Check sheet for the modelled part. Datum: model origin and axes. Units: mm. A direction names the side the tool comes from. Give positions to 0.01 mm unless a question says otherwise; leave off trailing zeros. Order: outer loops, then holes, each group sorted by start corner. A loop starts at its lowest first (then second) coordinate and runs counter-clockwise, first axis right, second up.
```python
from build123d import *

# Parameters (mm, degrees)
SKETCH_R      = 19
SKETCH_R_2    = 4
PAD_DEPTH     = 2
SKETCH001_R   = 15
SKETCH001_R_2 = 4
PAD001_DEPTH  = 1.4
SKETCH002_W   = 8.5
SKETCH002_H   = 8.5
POCKET_DEPTH  = 6


with BuildPart() as part:
    # Sketch → Pad (new body)
    with BuildSketch(Plane.XY):
        Circle(SKETCH_R)
        Circle(SKETCH_R_2, mode=Mode.SUBTRACT)
    extrude(amount=PAD_DEPTH)

    # Sketch001 (on Face4 of Pad) → Pad001 (join)
    with BuildSketch(Plane.XY.offset(2)):
        Circle(SKETCH001_R)
        Circle(SKETCH001_R_2, mode=Mode.SUBTRACT)
    extrude(amount=PAD001_DEPTH)

    # Sketch002 (on Face7 of Pad001) → Pocket (cut)
    with BuildSketch(Plane.XY.offset(3.4)):
        Rectangle(SKETCH002_W, SKETCH002_H)
    extrude(amount=-POCKET_DEPTH, mode=Mode.SUBTRACT)


solid = part.part
```
(1) Cross-section at D-D on x = 7.5. Enter the section's corners in (y, z), then the cut area to 3 significant figures.
Response values:
outline: (-17.46, 0) - (17.46, 0) - (17.46, 2) - (12.99, 2) - (12.99, 3.4) - (-12.99, 3.4) - (-12.99, 2) - (-17.46, 2) - close
area: 106 mm2
(2) Set-up check for faces 1 (the face through (-14.985, 0.66, 2.69)), 2 (the face through (-0.3, 4.5, 0)), 3 (the face through (4.25, 0, 2)): record each of +Z, -Z, +X, -X, +Y, -Y from which the full face is reachable in a straight line by a thin tool's end or side.
Response values:
face 1: +Z
face 2: -Z, +X, -X, +Y, -Y
face 3: +Z, -Z
(3) Cross-section at A-A on y = 0. Enter the section's corners in (x, z), then the cut area to 3 significant figures.
Response values:
outline: (-19, 0) - (-4.25, 0) - (-4.25, 3.4) - (-15, 3.4) - (-15, 2) - (-19, 2) - close; (4.25, 0) - (19, 0) - (19, 2) - (15, 2) - (15, 3.4) - (4.25, 3.4) - close
area: 89.1 mm2
(4) Material ranges on L1, parallel to X at y = 0.5, z = 0.7; L2, parallel to X at y = 3, z = 1; L3, parallel to Z at x = -17, y = 6, recorded low to high.
Response values:
L1: x = -18.99 to -4.25, 4.25 to 18.99
L2: x = -18.76 to -4.25, 4.25 to 18.76
L3: z = 0 to 2
(5) Cross-section at C-C on z = 0.7. Enter the section's corners in (x, y), then the cut area to 3 significant figures.
Response values:
outline: circle Ø38 at (0, 0); hole (-4.25, -4.25) - (4.25, -4.25) - (4.25, 4.25) - (-4.25, 4.25) - close
area: 1,060 mm2
(6) Release check for a two-part mould opening along X. For faces 4 (the face through (8.767, -16.856, 0.986)), 5 (the face through (-4.25, 0, 2)), 6 (the face through (14, 6, 2)), 7 (the face through (0, 4.25, 2)) record: released by +X, released by -X, zero draft, split by the parting line, or undercut.
Response values:
face 4: split by the parting line
face 5: undercut
face 6: zero draft
face 7: undercut
(7) Gauge pin test, flat ends, axial feed: pin 1 Ø1 at (x, z) = (12, 1.5) entering from -Y; pin 2 Ø1.5 at (x, z) = (-6, 2.5) entering from -Y; pin 3 Ø1.7 at (y, z) = (1.5, 1.5) entering from +X. Record the tip position at first contact, or that the pin passes through.
Response values:
pin 1: stops at y = -15.12
pin 2: stops at y = -18.2
pin 3: stops at x = 18.99
